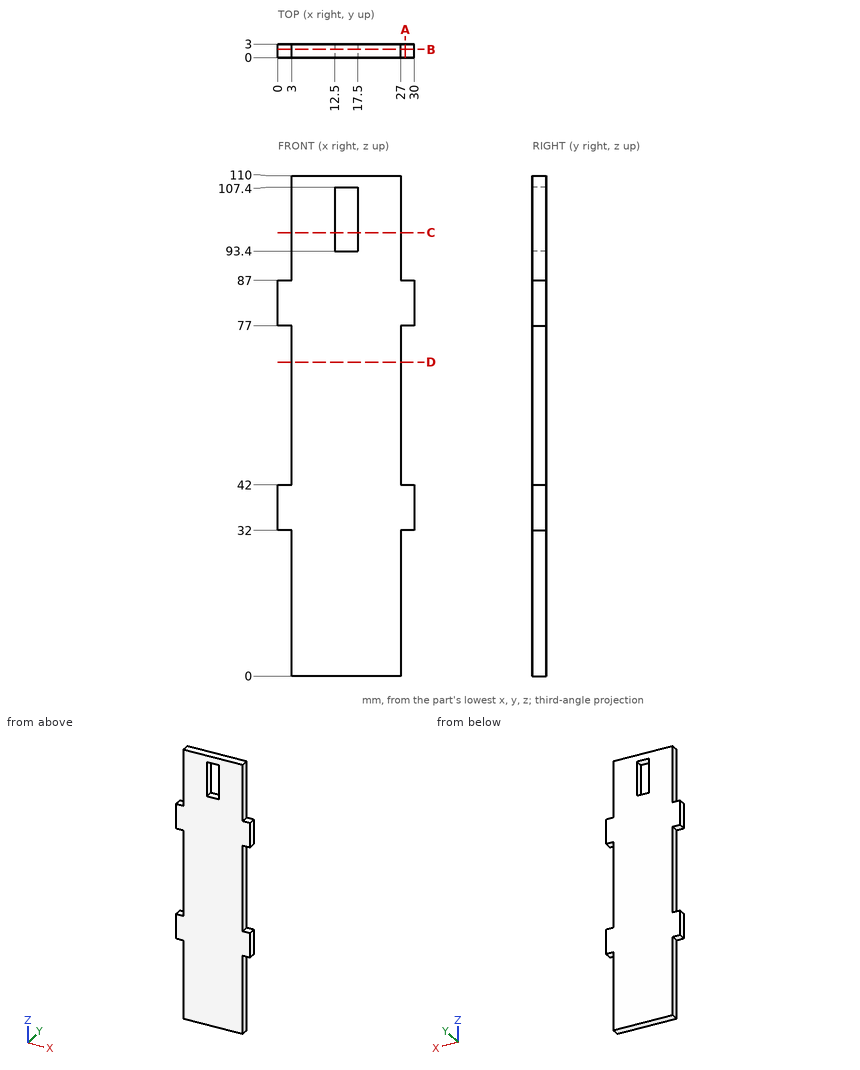
Geometry check sheet. Reference: drawing and pictorial views, mm from the part's lowest x, y, z. Round coordinates to 2 decimals unless told otherwise and drop trailing zeros. Loops run counter-clockwise (first coordinate to the right, second up) from the corner with the lowest first, then second, coordinate; pieces in that order, holes last. Notation, with made-up numbers: (19.5, 14) - (69.5, 14) arc R23 cw to (69.5, 43) - close; hole circle Ø10 at (23.25, 29). An arc over 180 degrees is marked (long way). One line per question, with ' | ' between items. Start each with the question number.
1. Depth check by flat-ended pin: pin 1 (1 mm diameter, centred on y = 0.5, z = 97, fed in from +X); pin 2 (1.5 mm diameter, centred on x = 2, y = 1, fed in from +Z); pin 3 (1.5 mm diameter, centred on y = 2, z = 104, fed in from -X). Enter the tip coordinate at first touch or a pass-through.
2. Cross-section at A-A on x = 28. Record the cut outline in (y, z), then the cut area to 3 significant figures.
3. Cross-section at D-D on z = 69. Record the cut outline in (x, y), then the cut area to 3 significant figures.
4. Scan lines: line 1 (Z direction, x = 1.5, y = 1); line 2 (X direction, y = 2.25, z = 99); line 3 (X direction, y = 2.85, z = 45). Record each from-to range of solid material in increasing order. Write a range as [from, to].
5. Cross-section at C-C on z = 97.5. Record the cut outline in (x, y).
6. Cross-section at B-B on y = 1.8. Record the cut outline in (x, z), then the cut area to 3 significant figures.
Taken from the geometry:
1) pin 1: x = 27 | pin 2: z = 87 | pin 3: x = 3
2) outline: (0, 32) - (3, 32) - (3, 42) - (0, 42) - close; (0, 77) - (3, 77) - (3, 87) - (0, 87) - close | area: 60.0 mm²
3) outline: (3, 0) - (27, 0) - (27, 3) - (3, 3) - close | area: 72.0 mm²
4) line 1: [32, 42], [77, 87] | line 2: [3, 12.5], [17.5, 27] | line 3: [3, 27]
5) outline: (3, 0) - (12.5, 0) - (12.5, 3) - (3, 3) - close; (17.5, 0) - (27, 0) - (27, 3) - (17.5, 3) - close
6) outline: (0, 32) - (3, 32) - (3, 0) - (27, 0) - (27, 32) - (30, 32) - (30, 42) - (27, 42) - (27, 77) - (30, 77) - (30, 87) - (27, 87) - (27, 110) - (3, 110) - (3, 87) - (0, 87) - (0, 77) - (3, 77) - (3, 42) - (0, 42) - close; hole (12.5, 93.4) - (17.5, 93.4) - (17.5, 107.4) - (12.5, 107.4) - close | area: 2,690 mm²
